Geometry: final body of the model. Coordinates: model frame, mm. A direction names the side the tool comes from. Round coordinates to 2 decimals unless told otherwise and drop trailing zeros. Loops run counter-clockwise (first coordinate to the right, second up) from the corner with the lowest first, then second, coordinate; pieces in that order, holes last. Notation, with made-up numbers: (-13.75, 4.5) - (19.25, 4.5) arc R28 cw to (19.25, 34.5) - close; hole circle Ø8 at (76, 54.25). An arc over 180 degrees is marked (long way). Answer as CSV lines item,"result".
Autodesk Inventor part; units mm, degrees
ref_plane "Work Plane1" through (12.75, -18.65, 0) normal (-0.2534, 0, 0.9674) x (0, 1, 0)
ref_plane "YZ Plane" through (0, 0, 0) normal (1, 0, 0) x (0, 1, 0)
ref_plane "XZ Plane" through (0, 0, 0) normal (0, 1, 0) x (-1, 0, 0)
sketch "Sketch1" plane through (0, 0, 0) normal (0, 0, 1) x (1, 0, 0)
  line L0 (-8.25, -14.15) -> (8.25, -14.15)
  line L1 (8.25, -14.15) -> (8.25, 14.15)
  line L2 (8.25, 14.15) -> (-8.25, 14.15)
  line L3 (-8.25, 14.15) -> (-8.25, -14.15)
  line L4 (-8.25, -14.15) -> (8.25, 14.15) construction
  line L5 (8.25, -14.15) -> (-8.25, 14.15) construction
  line L6 (-12.75, -18.65) -> (12.75, -18.65)
  line L7 (12.75, -18.65) -> (12.75, 18.65)
  line L8 (12.75, 18.65) -> (-12.75, 18.65)
  line L9 (-12.75, 18.65) -> (-12.75, -18.65)
  point P0 (0, 0)
  dimension "d0" = 16.5
  dimension "d1" = 28.3
  dimension "d2" = 4.5
extrude "Extrusion1" add sketch "Sketch1" along normal blind 15
ref_plane "Work Plane1" through (12.75, -18.65, 0) normal (-0.2534, 0, 0.9674) x (0, 1, 0)
sketch "Sketch2" plane through (12.75, -18.65, 0) normal (-0.2534, 0, 0.9674) x (0, 1, 0)
  line L0 (37.3, 0) -> (37.3, 24.6676) construction
  line L1 (37.3, 0) -> (0, 0)
  line L2 (0, 0) -> (0, -20)
  line L3 (0, -20) -> (37.3, -20)
  line L4 (37.3, -20) -> (37.3, 0)
  point P0 (18.65, 12.3338)
  dimension "d6" = 20
extrude "Extrusion2" add sketch "Sketch2" along normal blind 3
sketch "Sketch5" plane through (12.75, -18.65, 0) normal (0.2534, 0, -0.9674) x (-0.9674, 0, -0.2534)
  line L0 (-35, 24.95) -> (-5, 24.95)
  line L1 (-5, 24.95) -> (-5, 12.35)
  line L2 (-5, 12.35) -> (-35, 12.35)
  line L3 (-35, 12.35) -> (-35, 24.95)
  line L4 (-20, 0) -> (-20, 37.3) construction
  line L5 (-35, 24.95) -> (-5, 12.35) construction
  line L6 (-5, 24.95) -> (-35, 12.35) construction
  point P0 (12.3338, 18.65)
  point P1 (-20, 18.65)
  dimension "d15" = 30
  dimension "d16" = 12.6
extrude "Extrusion5" cut sketch "Sketch5" against normal blind 3
sketch "Sketch6" plane through (12.75, -18.65, 0) normal (0.2534, 0, -0.9674) x (-0.9674, 0, -0.2534)
  line L0 (0, 0) -> (-20, 0) construction
  line L1 (-20, 37.3) -> (0, 37.3) construction
  line L2 (-5, 24.95) -> (-20, 24.95) construction
  line L3 (-20, 12.35) -> (-5, 12.35) construction
  arc A0 (-20, 12.35) -> (0, 0) centre (0, 22.3693) ccw
  line L4 (-20, 0) -> (0, 0)
  line L5 (-20, 37.3) -> (-20, 24.95)
  line L6 (-20, 12.35) -> (-20, 0)
  arc A1 (0, 37.3) -> (-20, 24.95) centre (0, 14.9307) ccw
  line L7 (-20, 37.3) -> (-0.7859, 37.3) construction
  line L8 (0, 37.3) -> (-20, 37.3)
  point P0 (12.3338, 18.65)
  point P1 (0, 0)
extrude "Extrusion6" cut sketch "Sketch6" against normal blind 3
properties part number "Servo front rightleft holder"
(1) Section D-D (y = 12). Output: boundary loops of the cut face in (x, z), and give its area (3 significant figures).
Findings below:
outline,"(-12.75, 0) - (-8.25, 0) - (-8.25, 15) - (-12.75, 15) - close; (8.25, 0) - (12.75, 0) - (28.15, 4.03) - (27.39, 6.93) - (12.75, 3.1) - (12.75, 15) - (8.25, 15) - close"
area,"182 mm2"
(2) Draft query along Y for faces 6 (the face through (25, 6.3, 5)), 7 (the face through (-9, 0, 15)), 8 (the face through (0, -14.15, 7)), 9 (the face through (23.89, -15.22, 4.45)). Return one class per face: pulls with the +Y half, pulls with the -Y half, needs draft (parallel to the pull), parting line crosses it, or undercut.
Findings below:
face 6,"undercut"
face 7,"needs draft"
face 8,"undercut"
face 9,"pulls with the -Y half"
(3) Pin query (flat end, axial travel): P1, Ø4.5, axis at y = 2.5, z = 4.5, coming from the +X side; P2, Ø2, axis at y = -4, z = 12.5, coming from the +X side; P3, Ø2, axis at x = 20.5, y = 5.5, coming from the +Z side. Return the tip coordinate at first contact, or that it passes through.
Findings below:
P1,"x = 17.33"
P2,"x = 12.75"
P3,"z = 5.29"
(4) Access query for faces 1 (the face through (15.8, -0.3, 0.8)), 2 (the face through (12.75, 0, 9)), 3 (the face through (17.21, 0.09, 2.7)), 4 (the face through (-12.75, 0, 7)), 5 (the face through (-8.25, 0, 7)). Directions: +Z, -Z, +X, -X, +Y, -Y. A direction counts if a zero-diameter tool reaches every point of the face in a straight line with its end or side. Return the directions, or none.
Findings below:
face 1,"-Z, +X, +Y, -Y"
face 2,"+Z, +Y, -Y"
face 3,"+Z, +X"
face 4,"+Z, -Z, -X, +Y, -Y"
face 5,"+Z, -Z"
(5) Section B-B (z = 12). Output: boundary loops of the cut face in (x, y).
Findings below:
outline,"(-12.75, -18.65) - (12.75, -18.65) - (12.75, 18.65) - (-12.75, 18.65) - close; hole (-8.25, -14.15) - (8.25, -14.15) - (8.25, 14.15) - (-8.25, 14.15) - close"
(6) Material intervals for line 1 along Y through (x, z) = (2.5, 12.75); line 2 along X through (y, z) = (0, 4.5); line 3 along X through (y, z) = (-2.5, 3), sorted ascending.
Findings below:
line 1,"-18.65 to -14.15, 14.15 to 18.65"
line 2,"-12.75 to -8.25, 8.25 to 12.75"
line 3,"-12.75 to -8.25, 8.25 to 17.13"
(7) Section C-C (x = 5). Output: boundary loops of the cut face in (y, z).
Findings below:
outline,"(-18.65, 0) - (-14.15, 0) - (-14.15, 15) - (-18.65, 15) - close; (14.15, 0) - (18.65, 0) - (18.65, 15) - (14.15, 15) - close"
(8) Section A-A (y = 4). Output: boundary loops of the cut face in (x, z), and give its area (3 significant figures).
Findings below:
outline,"(-12.75, 0) - (-8.25, 0) - (-8.25, 15) - (-12.75, 15) - close; (8.25, 0) - (12.75, 0) - (17.59, 1.27) - (16.83, 4.17) - (12.75, 3.1) - (12.75, 15) - (8.25, 15) - close"
area,"149 mm2"
